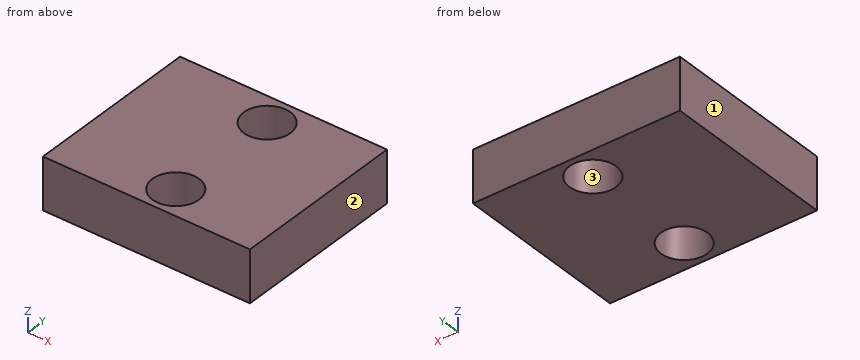
from build123d import *

# Parameters (mm, degrees)
CYLINDER001_R     = 1.8
CYLINDER001_DEPTH = 50
ARRAY001_Y_COUNT  = 2
ARRAY001_Y_PITCH  = 9
BOX002_W          = 16
BOX002_H          = 13.5
BOX002_DEPTH      = 4


with BuildPart() as array001:
    # Cylinder001 → Cylinder001 (new body)
    with BuildSketch(Plane(origin=(8.5, 2.25, -10), x_dir=(1, 0, 0), z_dir=(0, 0, 1))):
        Circle(CYLINDER001_R)
    extrude(amount=CYLINDER001_DEPTH)

    # Array001 Y: Array001 ×2


with BuildPart() as array001_1:
    add(array001.part)
    with Locations(*[(0, i * ARRAY001_Y_PITCH, 0) for i in range(1, ARRAY001_Y_COUNT)]):
        add(array001.part)


with BuildPart() as cut001:
    # Box002 → Box002 (new body)
    with BuildSketch(Plane.XY):
        with Locations((8, 6.75)):
            Rectangle(BOX002_W, BOX002_H)
    extrude(amount=BOX002_DEPTH)

    # Cut001: cut Array001
    add(array001_1.part, mode=Mode.SUBTRACT)


solid = cut001.part
Can you work these out from the model? Positions are in its coordinate system, mm. Face numbers are marked on the shaded views. Round coordinates to 2 decimals unless told otherwise and drop trailing zeros. Order: outer loops, then holes, each group sorted by start corner. A loop starts at its lowest first (then second) coordinate and runs counter-clockwise, first axis right, second up. Notation, with made-up numbers: (-38.75, 49.25) -> (-20.75, 49.25) arc R31 cw to (-20.75, 75.25) -> close; hole circle Ø2 at (34, -29). An arc over 180 degrees is marked (long way). Write each question's results on one line, items separated by ' | '. Start each with the question number.
Item 1: If we section it at C-C, the plane z = 2.9: Write out the boundary of the cut face in (x, y), then the cut area to 3 significant figures.
Item 2: If we section it at D-D, the plane y = 10.5: Write out the boundary of the cut face in (x, z).
Item 3: If we section it at A-A, the plane x = 8.5: Write out the boundary of the cut face in (y, z), then the cut area to 3 significant figures.
Item 4: Please list where these lines run through material, in increasing order: L1, parallel to Y at x = 8.5, z = 1.5; L2, parallel to X at y = 1.75, z = 3.75; L3, parallel to X at y = 11, z = 3.15.
Item 5: Thinking about a two-plate mould opening in X: for the marked faces 1, 2 and 3, which applies, +X half, -X half, draft (parallel to the pull), parting line (faces both ways), or undercut?
Item 6: Will this pin go through, and if not, where does the flat tip stop? pin 1 (2 mm diameter, centred on x = 8.5, y = 11.25, fed in from -Z).
Item 7: If we section it at B-B, the plane y = 2.25: Write out the boundary of the cut face in (x, z), then the cut area to 3 significant figures.
Results:
1) outline: (0, 0) -> (16, 0) -> (16, 13.5) -> (0, 13.5) -> close; hole circle Ø3.6 at (8.5, 2.25); hole circle Ø3.6 at (8.5, 11.25) | area: 196 mm2
2) outline: (0, 0) -> (6.86, 0) -> (6.86, 4) -> (0, 4) -> close; (10.14, 0) -> (16, 0) -> (16, 4) -> (10.14, 4) -> close
3) outline: (0, 0) -> (0.45, 0) -> (0.45, 4) -> (0, 4) -> close; (4.05, 0) -> (9.45, 0) -> (9.45, 4) -> (4.05, 4) -> close; (13.05, 0) -> (13.5, 0) -> (13.5, 4) -> (13.05, 4) -> close | area: 25.2 mm2
4) L1: y = 0 to 0.45, 4.05 to 9.45, 13.05 to 13.5 | L2: x = 0 to 6.77, 10.23 to 16 | L3: x = 0 to 6.72, 10.28 to 16
5) face 1: -X half | face 2: +X half | face 3: undercut
6) pin 1: passes through
7) outline: (0, 0) -> (6.7, 0) -> (6.7, 4) -> (0, 4) -> close; (10.3, 0) -> (16, 0) -> (16, 4) -> (10.3, 4) -> close | area: 49.6 mm2
